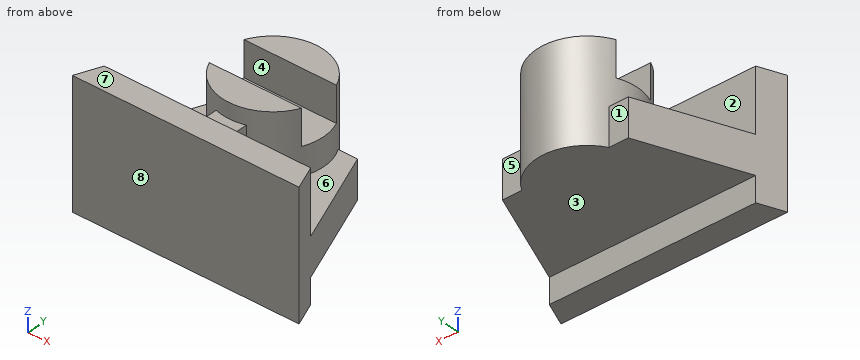
```python
from build123d import *

# Parameters (mm, degrees)
BOSS_EXTRUDE1_DEPTH      = 40
BOSS_EXTRUDE1_DEPTH_BACK = 10
BOSS_EXTRUDE2_DEPTH      = 15
BOSS_EXTRUDE3_DEPTH      = 34
SKETCH1_6_R              = 20
BOSS_EXTRUDE4_DEPTH      = 40
CUT_EXTRUDE1_DEPTH       = 14


with BuildPart() as part:
    # Sketch1 → Boss-Extrude1 (new, two sides: drawn at the far end of the back side and taken through both)
    with BuildSketch(Plane.XY.offset(-BOSS_EXTRUDE1_DEPTH_BACK)):
        Polygon((-60.696298415, -22.477026296), (-64.696298415, -32.477026296), (-44.696298415, -32.477026296), (-25.696298415, -32.477026296), (-13.696298415, -32.477026296), (25.303701585, -32.477026296), (21.303701585, -22.477026296), (-13.696298415, -22.477026296), (-25.696298415, -22.477026296), align=None)
    extrude(amount=BOSS_EXTRUDE1_DEPTH + BOSS_EXTRUDE1_DEPTH_BACK)

    # Sketch1_3 → Boss-Extrude2 (add)
    with BuildSketch(Plane.XY):
        with BuildLine():
            Line((-44.696298415, 17.522973704), (-60.696298415, -22.477026296))
            Line((-60.696298415, -22.477026296), (-25.696298415, -22.477026296))
            Line((-25.696298415, -22.477026296), (-25.696298415, -11.555810324))
            ThreePointArc((-25.696298415, -11.555810324), (-38.33377261, 0.267316902), (-37.016806491, 17.522973704))
            Line((-37.016806491, 17.522973704), (-44.696298415, 17.522973704))
        make_face()
        with BuildLine():
            Line((-13.696298415, -11.555810324), (-13.696298415, -22.477026296))
            Line((-13.696298415, -22.477026296), (21.303701585, -22.477026296))
            Line((21.303701585, -22.477026296), (5.303701585, 17.522973704))
            Line((5.303701585, 17.522973704), (-2.375790339, 17.522973704))
            ThreePointArc((-2.375790339, 17.522973704), (-1.05882422, 0.267316902), (-13.696298415, -11.555810324))
        make_face()
    extrude(amount=BOSS_EXTRUDE2_DEPTH)

    # Sketch1_4 → Boss-Extrude3 (add)
    with BuildSketch(Plane.XY):
        with BuildLine():
            Line((-25.696298415, -11.555810324), (-25.696298415, -22.477026296))
            Line((-25.696298415, -22.477026296), (-13.696298415, -22.477026296))
            Line((-13.696298415, -22.477026296), (-13.696298415, -11.555810324))
            ThreePointArc((-13.696298415, -11.555810324), (-19.696298415, -12.477026296), (-25.696298415, -11.555810324))
        make_face()
    extrude(amount=BOSS_EXTRUDE3_DEPTH)

    # Sketch1_6 → Boss-Extrude4 (add)
    with BuildSketch(Plane.XY):
        with Locations(Location((-19.696298415, 7.522973704, 0), (0, 0, 150))):
            Circle(SKETCH1_6_R)
    extrude(amount=BOSS_EXTRUDE4_DEPTH)

    # Sketch2 → Cut-Extrude1 (cut)
    with BuildSketch(Plane.XY.offset(40)):
        with BuildLine():
            Line((-39.696298415, 15.522973704), (0.303701585, 15.522973704))
            ThreePointArc((0.303701585, 15.522973704), (8.303701585, 7.522973704), (0.303701585, -0.477026296))
            Line((0.303701585, -0.477026296), (-39.696298415, -0.477026296))
            ThreePointArc((-39.696298415, -0.477026296), (-47.696298415, 7.522973704), (-39.696298415, 15.522973704))
        make_face()
    extrude(amount=-CUT_EXTRUDE1_DEPTH, mode=Mode.SUBTRACT)


solid = part.part
```
Model file for the job. Use its own axes, mm. Face numbers are marked on the shaded views. A direction names the side the tool comes from. Coordinates: 2 decimals unless noted, no trailing zeros. Order: outer loops, then holes, each group sorted by start corner. A loop starts at its lowest first (then second) coordinate and runs counter-clockwise, first axis right, second up. Notation, with made-up numbers: (2.25, 17.25) -> (54.25, 17.25) arc R25 cw to (54.25, 45.25) -> close; hole circle Ø5 at (69.5, 69). An arc over 180 degrees is marked (long way). Answer as a JSON object with one key per item and string values. Group by question number.
1) Drill centre lines: L1, parallel to Y at x = -2.5, z = 31; L2, parallel to Y at x = -8, z = 35.5; L3, parallel to X at y = -19, z = 33. Where is each one in solid material? Low to high.
2) Pull direction Y, two halves, no side cores. Call the marked faces 5, 6, 7 and 8: +Y half, -Y half, draft (parallel to the pull), parting line (faces both ways), or undercut.
3) Cut at A-A, the plane z = 36.5. Write the cut outline in (x, y).
4) Which spindle directions (+Z, -Z, +X, -X, +Y, -Y) get a long thin tool onto all of the face, cutting with end or side? Do the marked faces 1, 2, 3 and 4. Say none if no direction does.
5) Cut at B-B, the plane z = 30.5. Write the cut outline in (x, y).
6) Flat gauge pins, fed straight in: pin 1 (10 mm diameter, centred on y = 15, z = 26, fed in from -X); pin 2 (3 mm diameter, centred on x = -37.5, z = -6, fed in from +Y); pin 3 (2 mm diameter, centred on x = -37, z = 34, fed in from +Y). Where does each tip first touch, or does it go through?
7) Cut at D-D, the plane y = -14. Write the cut outline in (x, z).
8) Cut at C-C, the plane x = 2.5. Write the cut outline in (y, z), then the cut area to 3 significant figures.
Check values:
{
 "1": {"L1": "y = -32.48 to -22.48, -2.69 to -0.48, 15.52 to 17.74", "L2": "y = -32.48 to -22.48, -8.7 to -0.48, 15.52 to 23.75", "L3": "x = -25.7 to -13.7"},
 "2": {"face 5": "+Y half", "face 6": "undercut", "face 7": "draft", "face 8": "-Y half"},
 "3": {"outline": "(-64.7, -32.48) -> (25.3, -32.48) -> (21.3, -22.48) -> (-60.7, -22.48) -> close; (-38.03, -0.48) arc R20 ccw to (-1.37, -0.48) -> close; (-38.03, 15.52) -> (-1.37, 15.52) arc R20 ccw to start"},
 "4": {"face 1": "+Z, -Z, -X, +Y", "face 2": "+Z", "face 3": "-Z, +X, -X, +Y", "face 4": "+Z, +X, -X"},
 "5": {"outline": "(-64.7, -32.48) -> (25.3, -32.48) -> (21.3, -22.48) -> (-13.7, -22.48) -> (-13.7, -11.56) arc R20 ccw to (-1.37, -0.48) -> (-38.03, -0.48) arc R20 ccw to (-25.7, -11.56) -> (-25.7, -22.48) -> (-60.7, -22.48) -> close; (-38.03, 15.52) -> (-1.37, 15.52) arc R20 ccw to start"},
 "6": {"pin 1": "stops at x = -39.54", "pin 2": "stops at y = -22.48", "pin 3": "stops at y = 19.11"},
 "7": {"outline": "(-57.31, 0) -> (17.91, 0) -> (17.91, 15) -> (-13.7, 15) -> (-13.7, 34) -> (-25.7, 34) -> (-25.7, 15) -> (-57.31, 15) -> close"},
 "8": {"outline": "(-32.48, -10) -> (-22.48, -10) -> (-22.48, 0) -> (17.52, 0) -> (17.52, 15) -> (-22.48, 15) -> (-22.48, 40) -> (-32.48, 40) -> close", "area": "1,100 mm²"}
}
